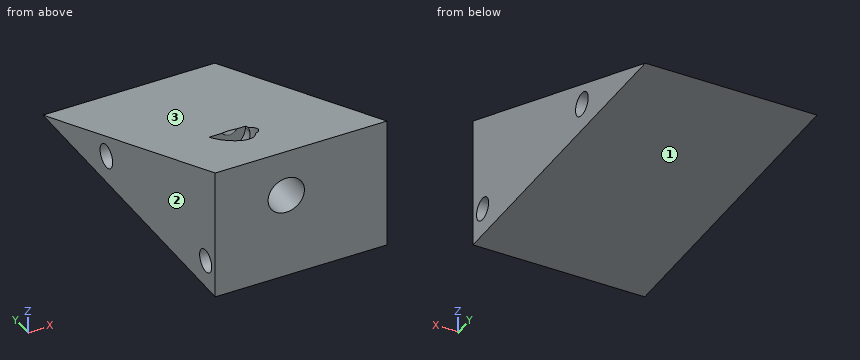
from build123d import *

# Parameters (mm, degrees)
F1_DEPTH = 25.4
F2_DEPTH = 12.192
F3_R     = 2.4676693698
F3_R_2   = 2.5740966664
F4_DEPTH = 43.18
F5_R     = 4.0713593192
F6_DEPTH = 9.144
F7_R     = 3.9791108566
F8_DEPTH = 24.13


with BuildPart() as f1:
    # F0 (on Right) → F1 (new body)
    with BuildSketch(Plane.YZ):
        Polygon((25.9079989046, 5.6388000958), (-44.5008017123, 34.5948003232), (-44.5008017123, 5.6388000958), align=None)
    extrude(amount=F1_DEPTH)

    # F2 (add): a face of the model
    f2_faces = [f1.faces().sort_by_distance(p)[0] for p in [
        (0, -21.0312015067, 15.2908001716),
    ]]
    extrude(f2_faces, amount=F2_DEPTH)

    # F3 (on face) → F4 (cut)
    with BuildSketch(Plane.YZ.offset(25.4)):
        with Locations((-40.5871495605, 11.6919511929)):
            Circle(F3_R)
        with Locations((0, 11.6919511929)):
            Circle(F3_R_2)
    extrude(amount=-F4_DEPTH, mode=Mode.SUBTRACT)

    # F5 (on face) → F6 (cut)
    with BuildSketch(Plane(origin=(0, 5.731464716, 13.9365089537), x_dir=(1, 0, 0), z_dir=(0, 0.3803470345, 0.9248438427))):
        with Locations((3.8493340835, -31.9517701864)):
            Circle(F5_R)
    extrude(amount=-F6_DEPTH, mode=Mode.SUBTRACT)

    # F7 (on face) → F8 (cut)
    with BuildSketch(Plane.XZ.offset(44.5008017123)):
        with Locations((3.3528024796, 24.3832562119)):
            Circle(F7_R)
    extrude(amount=-F8_DEPTH, mode=Mode.SUBTRACT)


solid = f1.part
Design review of the part built by this model. Coordinates are the model's own, in mm. Face numbers are marked on the shaded views. Round coordinates to 2 decimals unless told otherwise and drop trailing zeros. Write each loop counter-clockwise with the first axis right and the second up, starting at its lowest first coordinate (ties: lowest second). Pieces come first, ordered by that corner, then holes. Notation, with made-up numbers: (46, 44.5) - (92, 44.5) arc R29 ccw to (92, 71.5) - close; hole circle Ø2 at (83.5, -30). An arc over 180 degrees is marked (long way). Use a Markdown table: item, result. Add a question column.
1. We need section C-C (y = 0). State the section outline as (x, z) points, then the cut area to 3 significant figures.
2. We need section D-D (x = -8). State the section outline as (y, z) points, then the cut area to 3 significant figures.
3. Clearance check with flat-ended pins moving along their axes: pin 1 (6 mm diameter, centred on x = 16.5, z = 24.5, fed in from +Y); pin 2 (10.5 mm diameter, centred on x = 3.35, z = 24.38, fed in from +Y); pin 3 (8 mm diameter, centred on x = 16.5, y = -7, fed in from +Z); pin 4 (4 mm diameter, centred on y = 0, z = 11.69, fed in from +X). State where each tip first meets the part, or that it passes through.
4. Wall thickness on probe 1 along Y at (x, z) = (23, 10.5); probe 2 along X at (y, z) = (-22.5, 19.5); probe 3 along Y at (x, z) = (16, 9.5): over which ranges is each line inside the solid? List them lowest first.
5. We need section B-B (y = -40). State the section outline as (x, z) points.
6. We need section A-A (x = 3.5). State the section outline as (y, z) points, then the cut area to 3 significant figures.
7. Mouldability with a two-part tool opening along Z and no side actions: class the marked faces 1, 2 and 3 as +Z half, -Z half, draft (parallel to the pull), parting line (faces both ways), or undercut.
Output:
| question | item | result |
|---|---|---|
| 1 | outline | (-12.19, 5.64) - (25.4, 5.64) - (25.4, 9.12) - (-12.19, 9.12) - close; (-12.19, 14.27) - (25.4, 14.27) - (25.4, 16.29) - (-12.19, 16.29) - close |
| 1 | area | 207 mm2 |
| 2 | outline | (-44.5, 5.64) - (25.91, 5.64) - (-44.5, 34.59) - close; hole circle Ø4.94 at (-40.59, 11.69); hole circle Ø5.15 at (0, 11.69) |
| 2 | area | 979 mm2 |
| 3 | pin 1 | stops at y = -12.66 |
| 3 | pin 2 | stops at y = -6.9 |
| 3 | pin 3 | stops at z = 20.82 |
| 3 | pin 4 | passes through |
| 4 | probe 1 | y = -44.5 to -42.75, -38.43 to -2.28, 2.28 to 14.09 |
| 4 | probe 2 | x = -12.19 to 2.21, 5.49 to 25.4 |
| 4 | probe 3 | y = -44.5 to -41.72, -39.45 to -1.35, 1.35 to 16.52 |
| 5 | outline | (-12.19, 5.64) - (25.4, 5.64) - (25.4, 9.3) - (-12.19, 9.3) - close; (-12.19, 14.09) - (25.4, 14.09) - (25.4, 32.74) - (-12.19, 32.74) - close; hole circle Ø7.96 at (3.35, 24.38) |
| 6 | outline | (-44.5, 5.64) - (25.91, 5.64) - (-20.07, 24.55) - (-20.37, 23.81) - (-20.37, 20.41) - (-21.77, 20.41) - (-23.55, 16.09) - (-31.05, 19.18) - (-30.54, 20.41) - (-44.5, 20.41) - close; (-44.5, 28.36) - (-29.34, 28.36) - (-44.5, 34.59) - close; hole circle Ø4.94 at (-40.59, 11.69); hole circle Ø5.15 at (0, 11.69) |
| 6 | area | 780 mm2 |
| 7 | face 1 | -Z half |
| 7 | face 2 | draft |
| 7 | face 3 | +Z half |
